For this review, take the finished solid that the model builds, in its own axes (mm). Face numbers are marked on the shaded views. A direction names the side the tool comes from. Round coordinates to 2 decimals unless told otherwise and drop trailing zeros. Order: outer loops, then holes, each group sorted by start corner. A loop starts at its lowest first (then second) coordinate and runs counter-clockwise, first axis right, second up. Notation, with made-up numbers: (27, 12.25) -> (77, 12.25) arc R31 cw to (77, 49.25) -> close; hole circle Ø1 at (47, -18). An arc over 180 degrees is marked (long way). Put each result on its own line as item: value. Start each with the question number.
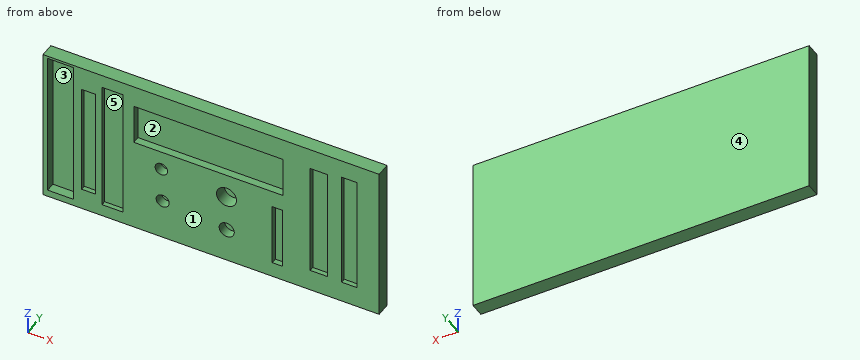
```python
from build123d import *

# Parameters (mm, degrees)
F0_W      = 457.2
F0_H      = 215.903491
F1_DEPTH  = 19.05
F2_W      = 20.6375
F2_H      = 161.925
F3_DEPTH  = 6.35
F4_W      = 23.8125
F4_H      = 157.1625
F5_DEPTH  = 6.35
F6_W      = 203.2
F6_H      = 55.5625
F7_DEPTH  = 10.16
F8_W      = 14.2875
F8_H      = 86.36
F9_DEPTH  = 7.62
F10_W     = 34.925
F10_H     = 203.2
F11_DEPTH = 12.7
F12_W     = 19.05
F12_H     = 153.9875
F13_DEPTH = 6.35
F14_R     = 13.6525
F15_DEPTH = 17.78
F16_R     = 10.287
F17_DEPTH = 12.7
F18_R     = 8.89
F19_DEPTH = 12.7
F20_R     = 8.509
F21_DEPTH = 12.7
F22_W     = 28.575
F22_H     = 180.975
F23_DEPTH = 6.35


with BuildPart() as f1:
    # F0 (on Front) → F1 (new body)
    with BuildSketch(Plane.XZ):
        with Locations((228.6, 107.951746)):
            Rectangle(F0_W, F0_H)
    extrude(amount=-F1_DEPTH)

    # F2 (on Front) → F3 (cut)
    with BuildSketch(Plane.XZ):
        with Locations((416.386539, 109.953294)):
            Rectangle(F2_W, F2_H)
    extrude(amount=-F3_DEPTH, mode=Mode.SUBTRACT)

    # F4 (on face) → F5 (cut)
    with BuildSketch(Plane.XZ):
        with Locations((375.281944, 108.470284)):
            Rectangle(F4_W, F4_H)
    extrude(amount=-F5_DEPTH, mode=Mode.SUBTRACT)

    # F6 (on face) → F7 (cut)
    with BuildSketch(Plane.XZ):
        with Locations((225.059846, 158.248464)):
            Rectangle(F6_W, F6_H)
    extrude(amount=-F7_DEPTH, mode=Mode.SUBTRACT)

    # F8 (on face) → F9 (cut)
    with BuildSketch(Plane.XZ):
        with Locations((318.874671, 64.148307)):
            Rectangle(F8_W, F8_H)
    extrude(amount=-F9_DEPTH, mode=Mode.SUBTRACT)

    # F10 (on face) → F11 (cut)
    with BuildSketch(Plane.XZ):
        with Locations((23.808912, 111.051154)):
            Rectangle(F10_W, F10_H)
    extrude(amount=-F11_DEPTH, mode=Mode.SUBTRACT)

    # F12 (on face) → F13 (cut)
    with BuildSketch(Plane.XZ):
        with Locations((62.019332, 106.47686)):
            Rectangle(F12_W, F12_H)
    extrude(amount=-F13_DEPTH, mode=Mode.SUBTRACT)

    # F14 (on face) → F15 (cut)
    with BuildSketch(Plane.XZ):
        with Locations((249.594485, 97.142791)):
            Circle(F14_R)
    extrude(amount=-F15_DEPTH, mode=Mode.SUBTRACT)

    # F16 (on face) → F17 (cut)
    with BuildSketch(Plane.XZ):
        with Locations((249.844001, 46.58331)):
            Circle(F16_R)
    extrude(amount=-F17_DEPTH, mode=Mode.SUBTRACT)

    # F18 (on face) → F19 (cut)
    with BuildSketch(Plane.XZ):
        with Locations((162.750646, 55.861603)):
            Circle(F18_R)
    extrude(amount=-F19_DEPTH, mode=Mode.SUBTRACT)

    # F20 (on face) → F21 (cut)
    with BuildSketch(Plane.XZ):
        with Locations((160.950046, 104.224064)):
            Circle(F20_R)
    extrude(amount=-F21_DEPTH, mode=Mode.SUBTRACT)

    # F22 (on face) → F23 (cut)
    with BuildSketch(Plane.XZ):
        with Locations((94.598287, 107.38296)):
            Rectangle(F22_W, F22_H)
    extrude(amount=-F23_DEPTH, mode=Mode.SUBTRACT)


solid = f1.part
```
Item 1: For L1, parallel to X at y = 7.25, z = 30.5; L2, parallel to X at y = 2, z = 21.5; L3, parallel to X at y = 2, z = 119.5, list the stretches that pass through material, from the lowest coordinate up.
Item 2: Mouldability with a two-part tool opening along X and no side actions: class the marked faces 3, 4 and 5 as +X half, -X half, draft (parallel to the pull), parting line (faces both ways), or undercut.
Item 3: Consider section B-B, the plane x = 179.5. Write out the cut boundary in (y, z), plus the area to 3 significant figures.
Item 4: Consider section A-A, the plane z = 71. Write out the cut boundary in (x, y), plus the area to 3 significant figures.
Item 5: Consider section C-C, the plane z = 154. Write out the cut boundary in (x, y).
Item 6: Insertion check: pin 1 Ø12 at (x, z) = (241, 146) entering from -Y; pin 2 Ø16 at (x, z) = (162.75, 55.86) entering from -Y; pin 3 Ø1 at (y, z) = (2, 119.5) entering from -X. Each pin has a flat end and moves straight along its axis. Give the tip position at first contact, or say it passes through.
Item 7: Tool access review of the marked faces 1 and 2: name each direction out of +Z, -Z, +X, -X, +Y, -Y from which nothing blocks a thin tool from reaching the whole face with its end or side.
Evaluation:
1. L1: x = 0 to 6.35, 41.27 to 311.73, 326.02 to 457.2
1. L2: x = 0 to 6.35, 41.27 to 80.31, 108.89 to 311.73, 326.02 to 457.2
1. L3: x = 0 to 6.35, 41.27 to 52.49, 71.54 to 80.31, 108.89 to 363.38, 387.19 to 406.07, 426.71 to 457.2
2. face 3: undercut
2. face 4: draft
2. face 5: undercut
3. outline: (0, 0) -> (19.05, 0) -> (19.05, 215.9) -> (0, 215.9) -> (0, 186.03) -> (10.16, 186.03) -> (10.16, 130.47) -> (0, 130.47) -> close
3. area: 3,550 mm^2
4. outline: (0, 0) -> (6.35, 0) -> (6.35, 12.7) -> (41.27, 12.7) -> (41.27, 0) -> (52.49, 0) -> (52.49, 6.35) -> (71.54, 6.35) -> (71.54, 0) -> (80.31, 0) -> (80.31, 6.35) -> (108.89, 6.35) -> (108.89, 0) -> (311.73, 0) -> (311.73, 7.62) -> (326.02, 7.62) -> (326.02, 0) -> (363.38, 0) -> (363.38, 6.35) -> (387.19, 6.35) -> (387.19, 0) -> (406.07, 0) -> (406.07, 6.35) -> (426.71, 6.35) -> (426.71, 0) -> (457.2, 0) -> (457.2, 19.05) -> (0, 19.05) -> close
4. area: 7,570 mm^2
5. outline: (0, 0) -> (6.35, 0) -> (6.35, 12.7) -> (41.27, 12.7) -> (41.27, 0) -> (52.49, 0) -> (52.49, 6.35) -> (71.54, 6.35) -> (71.54, 0) -> (80.31, 0) -> (80.31, 6.35) -> (108.89, 6.35) -> (108.89, 0) -> (123.46, 0) -> (123.46, 10.16) -> (326.66, 10.16) -> (326.66, 0) -> (363.38, 0) -> (363.38, 6.35) -> (387.19, 6.35) -> (387.19, 0) -> (406.07, 0) -> (406.07, 6.35) -> (426.71, 6.35) -> (426.71, 0) -> (457.2, 0) -> (457.2, 19.05) -> (0, 19.05) -> close
6. pin 1: stops at y = 10.16
6. pin 2: stops at y = 12.7
6. pin 3: stops at x = 0
7. face 1: +Z, -Z, +X, -X, -Y
7. face 2: -Y
